Solid Edge part; units mm, degrees
sketch "Sketch1" plane through (0, 0, 0) normal (0, -1, 0) x (1, 0, 0)
  line L0 (50, 0) -> (80, 0)
  line L1 (80, 0) -> (83.7743, 21.405)
  line L2 (145, -50) -> (103.7743, 21.405)
  line L3 (145, -50) -> (205, -50)
  line L4 (205, -50) -> (205, -34)
  line L5 (205, -34) -> (158.8564, -34)
  line L6 (158.8564, -34) -> (123.387, 27.4348)
  line L7 (123.387, 27.4348) -> (115, 75)
  line L8 (115, 75) -> (106.1714, 75)
  line L9 (100, 110) -> (106.1714, 75)
  line L10 (60, 110) -> (100, 110)
  line L11 (60, 90) -> (60, 110)
  line L12 (50, 90) -> (60, 90)
  line L13 (50, 0) -> (50, 90)
  arc A0 (83.7743, 21.405) -> (103.7743, 21.405) centre (93.7743, 21.405) cw
revolve "RevolvedProtrusion1" add sketch "Sketch1" angle 360 about axis through (0, 0, -50) along (0, 0, 1)
hole "Agujero_1" at (0, 80, 110) direction (0, 0, -1) diameter 12.376 depth 36 tip angle 118 thread major 14 thread length 20
pattern_circular "Pattern1" count 8 over 360 about axis through (0, 0, 0) along (0, 0, -1) of "Agujero_1"
hole "Agujero_10" at (180, 0, -34) direction (0, 0, -1) diameter 17.5 end up to next
pattern_circular "Pattern3" count 8 over 360 about axis through (0, 0, 0) along (0, 0, -1) of "Agujero_10"
sketch "Sketch2" plane through (0, 0, -34) normal (0, 0, 1) x (1, 0, 0)
  arc A0 (150.1515, 92.0844) -> (154.9884, 105.3736) centre (159.2146, 96.3105) cw
  line L0 (154.9884, 105.3736) -> (173.1145, 113.826)
  line L1 (180.3455, 50.9951) -> (198.4716, 59.4475)
  arc A1 (167.0562, 55.832) -> (180.3455, 50.9951) centre (176.1193, 60.0582) ccw
  line L2 (150.1515, 92.0844) -> (167.0562, 55.832)
extrude "VaciadoExtruido_1" cut sketch "Sketch2" against normal blind 16 material side at (149.8647, 99.7136, -34)
pattern_circular "Pattern5" count 8 over 360 about axis through (0, 0, 0) along (0, 0, -1) of "VaciadoExtruido_1"
Design review of the part built by this model. Coordinates are the model's own, in mm. A direction names the side the tool comes from. Coordinates: 2 decimals unless noted, no trailing zeros. Order: outer loops, then holes, each group sorted by start corner. A loop starts at its lowest first (then second) coordinate and runs counter-clockwise, first axis right, second up.
1) Take a section at B-B, the plane z = -23. Give the boundary of the cut face in (x, y).
2) Wall thickness on line 1 along Y through (x, z) = (-68.5, 14); line 2 along Y through (x, z) = (0, -46.5); line 3 along Y through (x, z) = (-180, -39.75): over which ranges is each line inside the solid? List them lowest first.
3) Mouldability with a two-part tool opening along Y and no side actions: class faces 5 (the flat face through (-109.08, 162.94, -41.89)), 6 (the flat face through (109.08, -162.94, -41.89)), 7 (the cylindrical face through (188.676, 1.139, -41.888)) as +Y half, -Y half, draft (parallel to the pull), parting line (faces both ways), or undercut.
4) For faces 1 (the cylindrical face through (172.6, 50.7, -41.9)), 2 (the flat face through (-164.54, 59.59, -41.89)), 3 (the flat face through (-192.347, 38.083, -41.888)), 4 (the cylindrical face through (-6.04, -81.34, 91.75)), list the 3-axis set-ups (+Z, -Z, +X, -X, +Y, -Y) from which the entire face can be reached by the end or side of a thin tool; tool diameter is ignored.
5) Take a section at A-A, the plane z = 56.5. Give the boundary of the cut face in (x, y).
6) Clearance check with flat-ended pins moving along their axes: pin 1 (10 mm diameter, centred on x = -85.5, z = -16, fed in from -Y); pin 2 (10 mm diameter, centred on x = -56.57, y = -56.57, fed in from -Z); pin 3 (10 mm diameter, centred on y = 125.5, z = -5, fed in from +X). State where each tip first meets the part, or that it passes through.
Returned:
1. outline: circle Ø305.01 at (0, 0); hole circle Ø258.82 at (0, 0)
2. line 1: y = -111.83 to -83.56, -45.92 to 45.92, 83.56 to 111.83
2. line 2: y = -205 to -188.75, -171.25 to -142.98, 142.98 to 171.25, 188.75 to 205
2. line 3: y = -50.84 to -8.75, 8.75 to 34.5, 97.44 to 98.11
3. face 5: +Y half
3. face 6: -Y half
3. face 7: undercut
4. face 1: +Z, -Z
4. face 2: +Z, -Z, -X
4. face 3: +Z, -Z, +Y
4. face 4: +Z
5. outline: circle Ø236.52 at (0, 0); hole circle Ø100 at (0, 0)
6. pin 1: stops at y = -126.23
6. pin 2: stops at z = 0
6. pin 3: stops at x = 77.01
